The model under review builds one solid part; all positions refer to its coordinate system, in mm. Face numbers are marked on the shaded views. A direction names the side the tool comes from. Coordinates: 2 decimals unless noted, no trailing zeros. Order: outer loops, then holes, each group sorted by start corner. A loop starts at its lowest first (then second) coordinate and runs counter-clockwise, first axis right, second up.
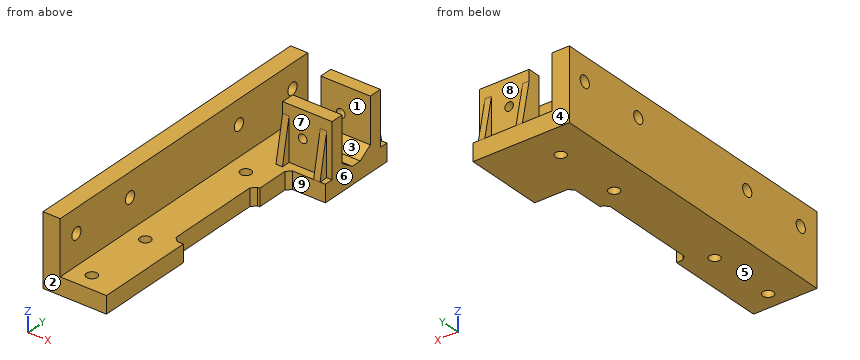
```python
from build123d import *

# Parameters (mm, degrees)
SKETCH1_W               = 24.51
SKETCH1_H               = 148
BOSS_EXTRUDE1_DEPTH     = 8
SKETCH2_W               = 8
SKETCH2_H               = 148
BOSS_EXTRUDE2_DEPTH     = 25
SKETCH4_W               = 20.3
SKETCH4_H               = 36.8
BOSS_EXTRUDE3_DEPTH     = 8
SKETCH5_W               = 23
SKETCH5_H               = 6
BOSS_EXTRUDE4_DEPTH     = 25
CUT_EXTRUDE2_REACH      = 151.752
SKETCH6_R               = 2
RIB1_REACH              = 159.03
SKETCH8_WALL_W          = 336.456302216
SKETCH8_WALL_H          = 3
MIRROR2_COPY_1_REACH    = 159.03
MIRROR2_COPY_1_SKETCH_W = 336.456302216
MIRROR2_COPY_1_SKETCH_H = 3
SKETCH3_R               = 2.5
CUT_EXTRUDE1_DEPTH      = 10
SKETCH12_R              = 2.75
CUT_EXTRUDE3_DEPTH      = 8
SKETCH13_W              = 5
SKETCH13_H              = 46
BOSS_EXTRUDE5_DEPTH     = 8
SKETCH14_W              = 3
SKETCH14_H              = 17
BOSS_EXTRUDE6_DEPTH     = 8
CHAMFER1_SIZE           = 2
CHAMFER2_SIZE           = 6
CHAMFER2_SIZE2          = 4.047051101


with BuildPart() as part:
    # Sketch1 → Boss-Extrude1 (new body)
    with BuildSketch(Plane.XY):
        with Locations((-12.255, 74)):
            Rectangle(SKETCH1_W, SKETCH1_H)
    extrude(amount=BOSS_EXTRUDE1_DEPTH)

    # Sketch2 → Boss-Extrude2 (add)
    with BuildSketch(Plane.XY.offset(8)):
        with Locations((-20.51, 74)):
            Rectangle(SKETCH2_W, SKETCH2_H)
    extrude(amount=BOSS_EXTRUDE2_DEPTH)

    # Sketch4 → Boss-Extrude3 (add)
    with BuildSketch(Plane(origin=(0, 0, 0), x_dir=(-1, 0, 0), z_dir=(0, 0, -1))):
        with Locations((-10.15, 129.6)):
            Rectangle(SKETCH4_W, SKETCH4_H)
    extrude(amount=-BOSS_EXTRUDE3_DEPTH)

    # Sketch5 → Boss-Extrude4 (add)
    with BuildSketch(Plane.XY.offset(8)):
        with Locations((8.8, 118.2)):
            Rectangle(SKETCH5_W, SKETCH5_H)
        with Locations((8.8, 141)):
            Rectangle(SKETCH5_W, SKETCH5_H)
    extrude(amount=BOSS_EXTRUDE4_DEPTH)

    # Cut-Extrude2: up to this face of the body (flat: up to its plane)
    cut_extrude2_end = Plane(part.part.faces().sort_by_distance((8.8, 115.2, 20.5))[0])
    # Sketch6 → Cut-Extrude2 (cut, up to the picked face)
    with BuildSketch(Plane(origin=(0, 144, 0), x_dir=(1, 0, 0), z_dir=(0, 1, 0)), mode=Mode.PRIVATE) as cut_extrude2_sk1:
        with Locations(Location((6.6, -20.5, 0), (0, 0, 270))):
            Circle(SKETCH6_R)
    cut_extrude2_tool1 = split(extrude(cut_extrude2_sk1.sketch, amount=-CUT_EXTRUDE2_REACH, mode=Mode.PRIVATE), bisect_by=cut_extrude2_end, keep=Keep.BOTH, mode=Mode.PRIVATE)
    add(cut_extrude2_tool1.solids().sort_by(Axis((6.6, 144, 20.5), (0, -1, 0)))[0], mode=Mode.SUBTRACT)

    # Sketch8 wall → Rib1 (add, up to next)
    with BuildSketch(Plane(origin=(16.3, 146, 18), x_dir=(0, -0.196116135138, 0.980580675691), z_dir=(0, -0.980580675691, -0.196116135138)), mode=Mode.PRIVATE) as rib1_sk1:
        Rectangle(SKETCH8_WALL_W, SKETCH8_WALL_H)
    rib1_tool1 = extrude(rib1_sk1.sketch, amount=RIB1_REACH, mode=Mode.PRIVATE) - part.part
    rib1 = rib1_tool1.solids().sort_by_distance((16.3, 146, 18))[0]
    add(rib1)

    # Mirror1: Rib1 across plane
    add(rib1.mirror(Plane.ZX.offset(129.6)))

    # Mirror2: Rib1 across plane
    add(rib1.mirror(Plane.ZY.offset(-7.55)))

    # Mirror2 copy 1 sketch → Mirror2 copy 1 (add, up to next)
    with BuildSketch(Plane(origin=(-1.2, 113.2, 18), x_dir=(0, 0.196116135138, 0.980580675691), z_dir=(0, 0.980580675691, -0.196116135138)), mode=Mode.PRIVATE) as mirror2_copy_1_sk1:
        Rectangle(MIRROR2_COPY_1_SKETCH_W, MIRROR2_COPY_1_SKETCH_H)
    mirror2_copy_1_tool1 = extrude(mirror2_copy_1_sk1.sketch, amount=MIRROR2_COPY_1_REACH, mode=Mode.PRIVATE) - part.part
    add(mirror2_copy_1_tool1.solids().sort_by_distance((-1.2, 113.2, 18))[0])

    # Sketch3 → Cut-Extrude1 (cut)
    with BuildSketch(Plane.XY.offset(8)):
        with Locations((-8, 8)):
            Circle(SKETCH3_R)
        with Locations((-8, 40)):
            Circle(SKETCH3_R)
        with Locations((-8, 100)):
            Circle(SKETCH3_R)
        with Locations((-8, 132)):
            Circle(SKETCH3_R)
    extrude(amount=-CUT_EXTRUDE1_DEPTH, mode=Mode.SUBTRACT)

    # Sketch12 → Cut-Extrude3 (cut)
    with BuildSketch(Plane.ZY.offset(24.51)):
        with Locations((22, 138.8)):
            Circle(SKETCH12_R)
        with Locations((22, 106.8)):
            Circle(SKETCH12_R)
        with Locations((22, 41.7)):
            Circle(SKETCH12_R)
        with Locations((22, 9.7)):
            Circle(SKETCH12_R)
    extrude(amount=-CUT_EXTRUDE3_DEPTH, mode=Mode.SUBTRACT)

    # Sketch13 → Boss-Extrude5 (add)
    with BuildSketch(Plane(origin=(0, 0, 0), x_dir=(-1, 0, 0), z_dir=(0, 0, -1))):
        with Locations((-2.5, 23)):
            Rectangle(SKETCH13_W, SKETCH13_H)
    extrude(amount=-BOSS_EXTRUDE5_DEPTH)

    # Sketch14 → Boss-Extrude6 (add)
    with BuildSketch(Plane(origin=(0, 0, 0), x_dir=(-1, 0, 0), z_dir=(0, 0, -1))):
        with Locations((-1.5, 102.7)):
            Rectangle(SKETCH14_W, SKETCH14_H)
    extrude(amount=-BOSS_EXTRUDE6_DEPTH)

    # Chamfer1
    chamfer1_edges = [part.edges().sort_by_distance(p)[0] for p in [
        (0, 46, 4),
        (3, 111.2, 4),
        (0, 94.2, 4),
    ]]
    chamfer(chamfer1_edges, length=CHAMFER1_SIZE)

    # Chamfer2
    chamfer2_edges = [part.edges().sort_by_distance(p)[0] for p in [
        (8.8, 121.2, 8),
        (8.8, 138, 8),
    ]]
    chamfer2_side = [part.faces().sort_by_distance(p)[0] for p in [
        (-4.974591741, 76.782250606, 8),
    ]]
    chamfer(chamfer2_edges, length=CHAMFER2_SIZE, length2=CHAMFER2_SIZE2, reference=chamfer2_side[0])


solid = part.part
```
(1) Draft analysis for pull direction Y (two halves, no side actions). For the marked faces 1, 2, 3 and 4, state which applies: released by +Y, released by -Y, zero draft, split by the parting line, or undercut.
A:
face 1: undercut
face 2: released by -Y
face 3: undercut
face 4: released by +Y
(2) We need section C-C, the plane x = -19.5. Write out the cut boundary in (y, z), and give its area (3 significant figures).
A:
outline: (0, 0) - (148, 0) - (148, 33) - (0, 33) - close; hole circle Ø5.5 at (9.7, 22); hole circle Ø5.5 at (41.7, 22); hole circle Ø5.5 at (106.8, 22); hole circle Ø5.5 at (138.8, 22)
area: 4,790 mm2
(3) Machinability: for the marked faces 5, 6, 7, 8 and 9, which of the approach directions +Z, -Z, +X, -X, +Y, -Y give a long, thin tool a straight path to every point of the face, cutting with its end or side? Answer none if there is none.
A:
face 5: -Z, +X, -X, +Y, -Y
face 6: +Z, -Z, +X, +Y, -Y
face 7: +Z, -Y
face 8: +Z, +Y
face 9: +Z, -Z, +X, -Y
(4) We need section D-D, the plane y = 76. Write out the cut boundary in (x, z).
A:
outline: (-24.51, 0) - (0, 0) - (0, 8) - (-16.51, 8) - (-16.51, 33) - (-24.51, 33) - close
(5) We need section B-B, the plane x = -8. Write out the cut boundary in (y, z), and give its area (3 significant figures).
A:
outline: (0, 0) - (5.5, 0) - (5.5, 8) - (0, 8) - close; (10.5, 0) - (37.5, 0) - (37.5, 8) - (10.5, 8) - close; (42.5, 0) - (97.5, 0) - (97.5, 8) - (42.5, 8) - close; (102.5, 0) - (129.5, 0) - (129.5, 8) - (102.5, 8) - close; (134.5, 0) - (148, 0) - (148, 8) - (134.5, 8) - close
area: 1,020 mm2
(6) Wall thickness on probe 1 along Y at (x, z) = (-8, 2.5); probe 2 along Y at (x, z) = (-19.5, 22); probe 3 along Y at (x, z) = (10.5, 31.5): over which ranges is each line inside the solid? List them lowest first.
A:
probe 1: y = 0 to 5.5, 10.5 to 37.5, 42.5 to 97.5, 102.5 to 129.5, 134.5 to 148
probe 2: y = 0 to 6.95, 12.45 to 38.95, 44.45 to 104.05, 109.55 to 136.05, 141.55 to 148
probe 3: y = 115.2 to 121.2, 138 to 144
(7) We need section A-A, the plane y = 106.8. Write out the cut boundary in (x, z).
A:
outline: (-24.51, 0) - (3, 0) - (3, 8) - (-16.51, 8) - (-16.51, 19.25) - (-24.51, 19.25) - close; (-24.51, 24.75) - (-16.51, 24.75) - (-16.51, 33) - (-24.51, 33) - close
(8) For pin 1 Ø6.5 at (y, z) = (99, 5.5) entering from +X; pin 2 Ø9 at (y, z) = (81, 5) entering from +X; pin 3 Ø2 at (y, z) = (113, 19) entering from +X, all flat-tipped, find the tip position at first contact; note any pin that passes through.
A:
pin 1: stops at x = 3
pin 2: stops at x = 0
pin 3: stops at x = 17.8
